from build123d import *

# Parameters (mm, degrees)
AUFSATZ_LINEAR_AUSTRAGEN1_DEPTH  = 10
SKIZZE2_R                        = 37.5
SKIZZE2_R_2                      = 27.5
AUFSATZ_LINEAR_AUSTRAGEN2_DEPTH  = 34
AUFSATZ_LINEAR_AUSTRAGEN3_DEPTH  = 35.4
SKIZZE4_W                        = 47.2
SKIZZE4_H                        = 42.2
SCHNITT_LINEAR_AUSTRAGEN1_DEPTH  = 178.743130331
SKIZZE8_W                        = 16.6
SKIZZE8_H                        = 30.2
SKIZZE8_W_2                      = 6.6
SKIZZE8_H_2                      = 20.2
AUFSATZ_LINEAR_AUSTRAGEN4_DEPTH  = 26.7
SCHNITT_LINEAR_AUSTRAGEN6_REACH  = 240.528
SKIZZE11_W                       = 45.873433193
SKIZZE11_H                       = 5
AUFSATZ_LINEAR_AUSTRAGEN5_DEPTH  = 26.7
SKIZZE12_W                       = 52.2
SKIZZE12_H                       = 52.2
SCHNITT_LINEAR_AUSTRAGEN7_DEPTH  = 8.7
SKIZZE13_W                       = 4
SKIZZE13_H                       = 52.2
AUFSATZ_LINEAR_AUSTRAGEN6_DEPTH  = 36.7
SCHNITT_LINEAR_AUSTRAGEN8_REACH  = 283.337
SKIZZE14_W                       = 42.2
SKIZZE14_H                       = 18.5
SKIZZE15_W                       = 52.2
SKIZZE15_H                       = 3
AUFSATZ_LINEAR_AUSTRAGEN7_DEPTH  = 36.7
VERRUNDUNG1_R                    = 3
SCHNITT_LINEAR_AUSTRAGEN9_REACH  = 202.455
SKIZZE16_R                       = 2.1
SKIZZE17_W                       = 33
SKIZZE17_H                       = 3
SCHNITT_LINEAR_AUSTRAGEN10_DEPTH = 11


with BuildPart() as part:
    # Skizze1 → Aufsatz-Linear austragen1 (new body)
    with BuildSketch(Plane(origin=(0, 0, 0), x_dir=(1, 0, 0), z_dir=(0, 1, 0))):
        with BuildLine():
            Line((-125, 26.1), (-125, -26.1))
            Line((-125, -26.1), (-53.866780115, -26.1))
            ThreePointArc((-53.866780115, -26.1), (-49.536653096, -28.6), (-49.536653096, -33.6))
            Line((-49.536653096, -33.6), (-85.103263039, -95.203175473))
            Line((-85.103263039, -95.203175473), (-39.896736961, -121.303175473))
            Line((-39.896736961, -121.303175473), (-4.330127019, -59.7))
            ThreePointArc((-4.330127019, -59.7), (0, -57.2), (4.330127019, -59.7))
            Line((4.330127019, -59.7), (39.896736961, -121.303175473))
            Line((39.896736961, -121.303175473), (85.103263039, -95.203175473))
            Line((85.103263039, -95.203175473), (49.536653096, -33.6))
            ThreePointArc((49.536653096, -33.6), (49.536653096, -28.6), (53.866780115, -26.1))
            Line((53.866780115, -26.1), (125, -26.1))
            Line((125, -26.1), (125, 26.1))
            Line((125, 26.1), (53.866780115, 26.1))
            ThreePointArc((53.866780115, 26.1), (49.536653096, 28.6), (49.536653096, 33.6))
            Line((49.536653096, 33.6), (85.103263039, 95.203175473))
            Line((85.103263039, 95.203175473), (39.896736961, 121.303175473))
            Line((39.896736961, 121.303175473), (4.330127019, 59.7))
            ThreePointArc((4.330127019, 59.7), (0, 57.2), (-4.330127019, 59.7))
            Line((-4.330127019, 59.7), (-39.896736961, 121.303175473))
            Line((-39.896736961, 121.303175473), (-85.103263039, 95.203175473))
            Line((-85.103263039, 95.203175473), (-49.536653096, 33.6))
            ThreePointArc((-49.536653096, 33.6), (-49.536653096, 28.6), (-53.866780115, 26.1))
            Line((-53.866780115, 26.1), (-125, 26.1))
        make_face()
    extrude(amount=AUFSATZ_LINEAR_AUSTRAGEN1_DEPTH)

    # Skizze2 → Aufsatz-Linear austragen2 (add)
    with BuildSketch(Plane(origin=(0, 10, 0), x_dir=(1, 0, 0), z_dir=(0, 1, 0))):
        with Locations(Location((0, 0, 0), (0, 0, 90))):
            Circle(SKIZZE2_R)
        with Locations(Location((0, 0, 0), (0, 0, 270))):
            Circle(SKIZZE2_R_2, mode=Mode.SUBTRACT)
    extrude(amount=AUFSATZ_LINEAR_AUSTRAGEN2_DEPTH)

    # Skizze3 → Aufsatz-Linear austragen3 (add)
    with BuildSketch(Plane(origin=(0, 10, 0), x_dir=(1, 0, 0), z_dir=(0, 1, 0))):
        Polygon((125, 26.1), (72.8, 26.1), (72.8, -26.1), (125, -26.1), (125, -21.1), (77.8, -21.1), (77.8, 21.1), (125, 21.1), align=None)
    extrude(amount=AUFSATZ_LINEAR_AUSTRAGEN3_DEPTH)

    # Skizze4 → Schnitt-Linear austragen1 (cut, through all)
    with BuildSketch(Plane(origin=(0, 10, 0), x_dir=(1, 0, 0), z_dir=(0, 1, 0))):
        with Locations((101.4, 0)):
            Rectangle(SKIZZE4_W, SKIZZE4_H)
    extrude(amount=-SCHNITT_LINEAR_AUSTRAGEN1_DEPTH, mode=Mode.SUBTRACT)

    # Skizze8 → Aufsatz-Linear austragen4 (add)
    with BuildSketch(Plane(origin=(0, 10, 0), x_dir=(1, 0, 0), z_dir=(0, 1, 0))):
        with Locations((-67, 10)):
            Rectangle(SKIZZE8_W, SKIZZE8_H)
        with Locations((-67, 10)):
            Rectangle(SKIZZE8_W_2, SKIZZE8_H_2, mode=Mode.SUBTRACT)
    extrude(amount=AUFSATZ_LINEAR_AUSTRAGEN4_DEPTH)

    # Schnitt-Linear austragen6: up to this face of the body (flat: up to its plane)
    schnitt_linear_austragen6_end = Plane(part.part.faces().sort_by_distance((-58.7, 23.35, -10))[0])
    # Skizze10 → Schnitt-Linear austragen6 (cut, up to the picked face)
    with BuildSketch(Plane.ZY.offset(75.3), mode=Mode.PRIVATE) as schnitt_linear_austragen6_sk1:
        with BuildLine():
            Line((-13.25, 34.2), (-13.25, 26.2))
            ThreePointArc((-13.25, 26.2), (-14.75, 24.7), (-16.25, 26.2))
            Line((-16.25, 26.2), (-16.25, 34.2))
            ThreePointArc((-16.25, 34.2), (-14.75, 35.7), (-13.25, 34.2))
        make_face()
    schnitt_linear_austragen6_tool1 = split(extrude(schnitt_linear_austragen6_sk1.sketch, amount=-SCHNITT_LINEAR_AUSTRAGEN6_REACH, mode=Mode.PRIVATE), bisect_by=schnitt_linear_austragen6_end, keep=Keep.BOTH, mode=Mode.PRIVATE)
    # Skizze10 → Schnitt-Linear austragen6 (cut, up to the picked face)
    with BuildSketch(Plane.ZY.offset(75.3), mode=Mode.PRIVATE) as schnitt_linear_austragen6_sk2:
        with BuildLine():
            Line((-3.75, 34.2), (-3.75, 26.2))
            ThreePointArc((-3.75, 26.2), (-5.25, 24.7), (-6.75, 26.2))
            Line((-6.75, 26.2), (-6.75, 34.2))
            ThreePointArc((-6.75, 34.2), (-5.25, 35.7), (-3.75, 34.2))
        make_face()
    schnitt_linear_austragen6_tool2 = split(extrude(schnitt_linear_austragen6_sk2.sketch, amount=-SCHNITT_LINEAR_AUSTRAGEN6_REACH, mode=Mode.PRIVATE), bisect_by=schnitt_linear_austragen6_end, keep=Keep.BOTH, mode=Mode.PRIVATE)
    # Skizze10 → Schnitt-Linear austragen6 (cut, up to the picked face)
    with BuildSketch(Plane.ZY.offset(75.3), mode=Mode.PRIVATE) as schnitt_linear_austragen6_sk3:
        with BuildLine():
            Line((-14, 14.5), (-6, 14.5))
            ThreePointArc((-6, 14.5), (-4.5, 13), (-6, 11.5))
            Line((-6, 11.5), (-14, 11.5))
            ThreePointArc((-14, 11.5), (-15.5, 13), (-14, 14.5))
        make_face()
    schnitt_linear_austragen6_tool3 = split(extrude(schnitt_linear_austragen6_sk3.sketch, amount=-SCHNITT_LINEAR_AUSTRAGEN6_REACH, mode=Mode.PRIVATE), bisect_by=schnitt_linear_austragen6_end, keep=Keep.BOTH, mode=Mode.PRIVATE)
    add(schnitt_linear_austragen6_tool1.solids().sort_by(Axis((-75.3, 30.2, -14.75), (1, 0, 0)))[0], mode=Mode.SUBTRACT)
    add(schnitt_linear_austragen6_tool2.solids().sort_by(Axis((-75.3, 30.2, -5.25), (1, 0, 0)))[0], mode=Mode.SUBTRACT)
    add(schnitt_linear_austragen6_tool3.solids().sort_by(Axis((-75.3, 13, -10), (1, 0, 0)))[0], mode=Mode.SUBTRACT)

    # Skizze11 → Aufsatz-Linear austragen5 (add)
    with BuildSketch(Plane(origin=(0, 10, 0), x_dir=(1, 0, 0), z_dir=(0, 1, 0))):
        with BuildLine():
            Line((-66.830127019, 105.753175473), (-58.169872981, 110.753175473))
            Line((-58.169872981, 110.753175473), (-14.252458915, 34.685982974))
            ThreePointArc((-14.252458915, 34.685982974), (-18.75, 32.475952642), (-22.912712953, 29.685982974))
            Line((-22.912712953, 29.685982974), (-66.830127019, 105.753175473))
        make_face()
        with BuildLine():
            Line((58.169872981, 110.753175473), (14.252458915, 34.685982974))
            ThreePointArc((14.252458915, 34.685982974), (18.75, 32.475952642), (22.912712953, 29.685982974))
            Line((22.912712953, 29.685982974), (66.830127019, 105.753175473))
            Line((66.830127019, 105.753175473), (58.169872981, 110.753175473))
        make_face()
        with BuildLine():
            Line((-58.169872981, -110.753175473), (-14.252458915, -34.685982974))
            ThreePointArc((-14.252458915, -34.685982974), (-18.75, -32.475952642), (-22.912712953, -29.685982974))
            Line((-22.912712953, -29.685982974), (-66.830127019, -105.753175473))
            Line((-66.830127019, -105.753175473), (-58.169872981, -110.753175473))
        make_face()
        with BuildLine():
            Line((66.830127019, -105.753175473), (58.169872981, -110.753175473))
            Line((58.169872981, -110.753175473), (14.252458915, -34.685982974))
            ThreePointArc((14.252458915, -34.685982974), (18.75, -32.475952642), (22.912712953, -29.685982974))
            Line((22.912712953, -29.685982974), (66.830127019, -105.753175473))
        make_face()
        with Locations((49.863283404, 23.6)):
            Rectangle(SKIZZE11_W, SKIZZE11_H)
        with Locations((49.863283404, -23.6)):
            Rectangle(SKIZZE11_W, SKIZZE11_H)
    extrude(amount=AUFSATZ_LINEAR_AUSTRAGEN5_DEPTH)

    # Skizze12 → Schnitt-Linear austragen7 (cut)
    with BuildSketch(Plane(origin=(0, 45.4, 0), x_dir=(1, 0, 0), z_dir=(0, 1, 0))):
        with Locations((98.9, 0)):
            Rectangle(SKIZZE12_W, SKIZZE12_H)
    extrude(amount=-SCHNITT_LINEAR_AUSTRAGEN7_DEPTH, mode=Mode.SUBTRACT)

    # Skizze13 → Aufsatz-Linear austragen6 (add)
    with BuildSketch(Plane(origin=(0, 36.7, 0), x_dir=(1, 0, 0), z_dir=(0, 1, 0))):
        with Locations((123, 0)):
            Rectangle(SKIZZE13_W, SKIZZE13_H)
    extrude(amount=-AUFSATZ_LINEAR_AUSTRAGEN6_DEPTH)

    # Schnitt-Linear austragen8: up to this face of the body (flat: up to its plane)
    schnitt_linear_austragen8_end = Plane(part.part.faces().sort_by_distance((72.8, 23.35, 0))[0])
    # Skizze14 → Schnitt-Linear austragen8 (cut, up to the picked face)
    with BuildSketch(Plane(origin=(125, 0, 0), x_dir=(0, 0, -1), z_dir=(1, 0, 0)), mode=Mode.PRIVATE) as schnitt_linear_austragen8_sk1:
        with Locations((0, 19.25)):
            Rectangle(SKIZZE14_W, SKIZZE14_H)
    schnitt_linear_austragen8_tool1 = split(extrude(schnitt_linear_austragen8_sk1.sketch, amount=-SCHNITT_LINEAR_AUSTRAGEN8_REACH, mode=Mode.PRIVATE), bisect_by=schnitt_linear_austragen8_end, keep=Keep.BOTH, mode=Mode.PRIVATE)
    add(schnitt_linear_austragen8_tool1.solids().sort_by(Axis((125, 19.25, 0), (-1, 0, 0)))[0], mode=Mode.SUBTRACT)

    # Skizze15 → Aufsatz-Linear austragen7 (add)
    with BuildSketch(Plane(origin=(0, 36.7, 0), x_dir=(1, 0, 0), z_dir=(0, 1, 0))):
        with Locations((98.9, 27.6)):
            Rectangle(SKIZZE15_W, SKIZZE15_H)
        with Locations((98.9, -27.6)):
            Rectangle(SKIZZE15_W, SKIZZE15_H)
    extrude(amount=-AUFSATZ_LINEAR_AUSTRAGEN7_DEPTH)

    # Verrundung1
    verrundung1_edges = [part.edges().sort_by_distance(p)[0] for p in [
        (72.8, 18.35, -26.1),
        (72.8, 18.35, 26.1),
    ]]
    fillet(verrundung1_edges, radius=VERRUNDUNG1_R - 0.0001)  # a hair under: the kernel refuses the full size

    # Schnitt-Linear austragen9: up to this face of the body (flat: up to its plane)
    schnitt_linear_austragen9_end = Plane(part.part.faces().sort_by_distance((98.9, 18.35, -29.1))[0])
    # Skizze16 → Schnitt-Linear austragen9 (cut, up to the picked face)
    with BuildSketch(Plane.XY.offset(29.1), mode=Mode.PRIVATE) as schnitt_linear_austragen9_sk1:
        with Locations((82.8, 24.7)):
            Circle(SKIZZE16_R)
    schnitt_linear_austragen9_tool1 = split(extrude(schnitt_linear_austragen9_sk1.sketch, amount=-SCHNITT_LINEAR_AUSTRAGEN9_REACH, mode=Mode.PRIVATE), bisect_by=schnitt_linear_austragen9_end, keep=Keep.BOTH, mode=Mode.PRIVATE)
    # Skizze16 → Schnitt-Linear austragen9 (cut, up to the picked face)
    with BuildSketch(Plane.XY.offset(29.1), mode=Mode.PRIVATE) as schnitt_linear_austragen9_sk2:
        with Locations((115, 24.7)):
            Circle(SKIZZE16_R)
    schnitt_linear_austragen9_tool2 = split(extrude(schnitt_linear_austragen9_sk2.sketch, amount=-SCHNITT_LINEAR_AUSTRAGEN9_REACH, mode=Mode.PRIVATE), bisect_by=schnitt_linear_austragen9_end, keep=Keep.BOTH, mode=Mode.PRIVATE)
    # Skizze16 → Schnitt-Linear austragen9 (cut, up to the picked face)
    with BuildSketch(Plane.XY.offset(29.1), mode=Mode.PRIVATE) as schnitt_linear_austragen9_sk3:
        with Locations((82.8, 4)):
            Circle(SKIZZE16_R)
    schnitt_linear_austragen9_tool3 = split(extrude(schnitt_linear_austragen9_sk3.sketch, amount=-SCHNITT_LINEAR_AUSTRAGEN9_REACH, mode=Mode.PRIVATE), bisect_by=schnitt_linear_austragen9_end, keep=Keep.BOTH, mode=Mode.PRIVATE)
    add(schnitt_linear_austragen9_tool1.solids().sort_by(Axis((82.8, 24.7, 29.1), (0, 0, -1)))[0], mode=Mode.SUBTRACT)
    add(schnitt_linear_austragen9_tool2.solids().sort_by(Axis((115, 24.7, 29.1), (0, 0, -1)))[0], mode=Mode.SUBTRACT)
    add(schnitt_linear_austragen9_tool3.solids().sort_by(Axis((82.8, 4, 29.1), (0, 0, -1)))[0], mode=Mode.SUBTRACT)

    # Skizze17 → Schnitt-Linear austragen10 (cut)
    with BuildSketch(Plane.XZ):
        with Locations((108.5, 27.6)):
            Rectangle(SKIZZE17_W, SKIZZE17_H)
        with Locations((108.5, -27.6)):
            Rectangle(SKIZZE17_W, SKIZZE17_H)
    extrude(amount=-SCHNITT_LINEAR_AUSTRAGEN10_DEPTH, mode=Mode.SUBTRACT)


solid = part.part
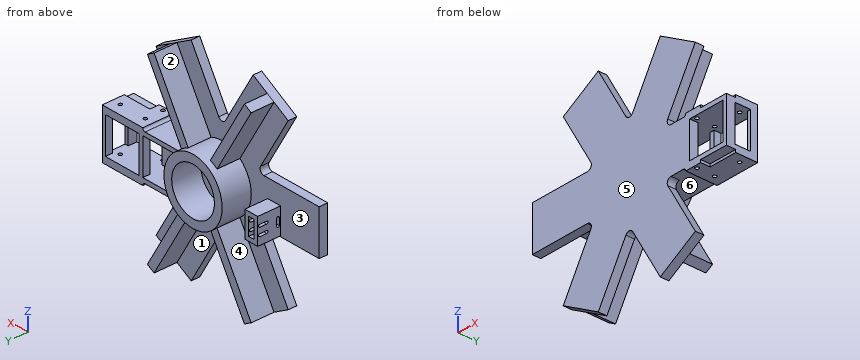
Can you work these out from the model? Positions are in its coordinate system, mm. Face numbers are marked on the shaded views. A direction names the side the tool comes from. Give positions to 0.01 mm unless a question says otherwise; leave off trailing zeros. Loops run counter-clockwise (first coordinate to the right, second up) from the corner with the lowest first, then second, coordinate; pieces in that order, holes last. Notation, with made-up numbers: M 0,43.5 L 55,43.5 A9 cw 55,54.5 Z; hole C 19,1.5 d9. An arc over 180 degrees is marked long. One line per item, written item: value. Start each with the question number.
1) If we section it at A-A, the plane x = 97: Write out the boundary of the cut face in (y, z), and give its area (3 significant figures).
2) Thinking about a two-plate mould opening in X: for the marked faces 4, 5 and 6, which applies, +X half, -X half, draft (parallel to the pull), parting line (faces both ways), or undercut?
3) If I drill on line 1 (Y direction, x = 82.8, z = -24.5); line 2 (Y direction, x = 82, z = 27); line 3 (Z direction, x = 110, y = 28), over which ranges is the centre line in solid material (lowest first)? Write a range as [from, to].
4) On a 3-axis mill with a long thin cutter (end or side, diameter ignored), from which of +Z, -Z, +X, -X, +Y, -Y can I reach the whole of each face in a straight line? I mean the marked faces 1, 2 and 3. Say none if no direction works.
5) If we section it at C-C, the plane y = 40.5: Write out the boundary of the cut face in (x, z), and give its area (3 significant figures).
6) If we section it at B-B, the plane z = -67: Write out the boundary of the cut face in (x, y), and give its area (3 significant figures).
7) I'm going to push flat-ended pins straight in: pin 1 (4 mm diameter, centred on x = -60.5, y = 32, fed in from +Z); pin 2 (5 mm diameter, centred on y = 25.5, z = 5, fed in from -X); pin 3 (2.5 mm diameter, centred on x = -74, y = 32, fed in from +Z). Where does each tip first touch, or does it pass through?
8) If we section it at D-D, the plane z = 43.5: Write out the boundary of the cut face in (x, y).
Completed:
1. outline: M 0,-26.1 L 11,-26.1 L 11,-29.1 L 36.7,-29.1 L 36.7,-21.1 L 0,-21.1 Z; M 0,21.1 L 36.7,21.1 L 36.7,29.1 L 11,29.1 L 11,26.1 L 0,26.1 Z
1. area: 521 mm^2
2. face 4: -X half
2. face 5: draft
2. face 6: undercut
3. line 1: y = [0, 1.9], [6.1, 22.6], [26.8, 36.7]
3. line 2: y = [0, 2.06], [5.94, 22.76], [26.64, 36.7]
3. line 3: z = [-29.1, -21.1], [21.1, 29.1]
4. face 1: -Z, +Y
4. face 2: +Z, +Y
4. face 3: +Y
5. outline: C 0,0 d75; hole C 0,0 d55
5. area: 2,040 mm^2
6. outline: M -68.82,0 L -8.54,0 L -8.54,10 L -32.91,10 L -32.91,36.7 L -44.46,36.7 L -44.46,10 L -68.82,10 Z; M 8.54,0 L 68.82,0 L 68.82,10 L 44.46,10 L 44.46,36.7 L 32.91,36.7 L 32.91,10 L 8.54,10 Z
6. area: 1,820 mm^2
7. pin 1: stops at z = 110.56
7. pin 2: stops at x = -75.3
7. pin 3: stops at z = 5.1
8. outline: M -55.25,0 L 55.25,0 L 55.25,10 L 30.89,10 L 30.89,36.7 L 19.34,36.7 L 19.34,10 L -19.34,10 L -19.34,36.7 L -30.89,36.7 L -30.89,10 L -55.25,10 Z
